from build123d import *

# Parameters (mm, degrees)
ESQUISSE2_W              = 92.64
ESQUISSE2_H              = 119.96
ESQUISSE2_W_2            = 88.74
ESQUISSE2_H_2            = 116.06
BASE_DEPTH               = 3
ESQUISSE3_R              = 4.5
SUPPORT_PCB_DEPTH        = 5
ESQUISSE4_R              = 2.25
ESQUISSE4_R_2            = 1.5
INSERT_M3_PCB_DEPTH      = 3
ESQUISSE4_3_R            = 1.5
PASSAGE_M3_PCB_DEPTH     = 5
ESQUISSE2_4_W            = 92.64
ESQUISSE2_4_H            = 119.96
ESQUISSE2_4_W_2          = 88.74
ESQUISSE2_4_H_2          = 116.06
WALLS_DEPTH              = 27
OUVERTURE_CONN_CMC_REACH = 133.396
ESQUISSE5_W              = 46.7
ESQUISSE5_H              = 20.1
CHANFREIN1_SIZE          = 12
CONG_1_R                 = 2
ESQUISSE6_R              = 2.25
INSERT_M3_BOX_DEPTH      = 3
ESQUISSE6_3_R            = 1.6
PASSAGE_M3_BOX_DEPTH     = 18
ESQUISSE10_R             = 3.1
BOSS_EXTRU_2_DEPTH       = 5
CONG_4_R                 = 5
PASSAGE_MAP_REACH        = 134.436
ESQUISSE11_R             = 3.5


with BuildPart() as part:
    # Esquisse2 → Base (new body)
    # profile 1 of 2: a face of its own
    with BuildSketch(Plane(origin=(0, 0, 0), x_dir=(1, 0, 0), z_dir=(0, 1, 0))):
        with Locations((0, 0.45)):
            Rectangle(ESQUISSE2_W, ESQUISSE2_H)
        with Locations((0, 0.45)):
            Rectangle(ESQUISSE2_W_2, ESQUISSE2_H_2, mode=Mode.SUBTRACT)
    # profile 2 of 2: a face of its own
    with BuildSketch(Plane(origin=(0, 0, 0), x_dir=(1, 0, 0), z_dir=(0, 1, 0))):
        with Locations((0, 0.45)):
            Rectangle(ESQUISSE2_W_2, ESQUISSE2_H_2)
    extrude(amount=-BASE_DEPTH)

    # Esquisse3 → Support_PCB (add)
    with BuildSketch(Plane(origin=(0, 0, 0), x_dir=(1, 0, 0), z_dir=(0, 1, 0))):
        with Locations(Location((-34.81, 28.71, 0), (0, 0, 270))):
            Circle(ESQUISSE3_R)
        with Locations(Location((34.79, 28.71, 0), (0, 0, 270))):
            Circle(ESQUISSE3_R)
        with Locations(Location((-19.57, -48, 0), (0, 0, 90))):
            Circle(ESQUISSE3_R)
        with Locations(Location((34.79, -48, 0), (0, 0, 90))):
            Circle(ESQUISSE3_R)
    extrude(amount=SUPPORT_PCB_DEPTH)

    # Esquisse4 → Insert_M3_PCB (cut)
    # profile 1 of 8: a face of its own
    with BuildSketch(Plane(origin=(0, 5, 0), x_dir=(1, 0, 0), z_dir=(0, 1, 0))):
        with Locations(Location((-34.81, 28.71, 0), (0, 0, 270))):
            Circle(ESQUISSE4_R)
        with Locations((-34.81, 28.71)):
            Circle(ESQUISSE4_R_2, mode=Mode.SUBTRACT)
    # profile 2 of 8: a face of its own
    with BuildSketch(Plane(origin=(0, 5, 0), x_dir=(1, 0, 0), z_dir=(0, 1, 0))):
        with Locations((-34.81, 28.71)):
            Circle(ESQUISSE4_R_2)
    # profile 3 of 8: a face of its own
    with BuildSketch(Plane(origin=(0, 5, 0), x_dir=(1, 0, 0), z_dir=(0, 1, 0))):
        with Locations(Location((34.79, 28.71, 0), (0, 0, 270))):
            Circle(ESQUISSE4_R)
        with Locations((34.79, 28.71)):
            Circle(ESQUISSE4_R_2, mode=Mode.SUBTRACT)
    # profile 4 of 8: a face of its own
    with BuildSketch(Plane(origin=(0, 5, 0), x_dir=(1, 0, 0), z_dir=(0, 1, 0))):
        with Locations((34.79, 28.71)):
            Circle(ESQUISSE4_R_2)
    # profile 5 of 8: a face of its own
    with BuildSketch(Plane(origin=(0, 5, 0), x_dir=(1, 0, 0), z_dir=(0, 1, 0))):
        with Locations(Location((34.79, -48, 0), (0, 0, 270))):
            Circle(ESQUISSE4_R)
        with Locations((34.79, -48)):
            Circle(ESQUISSE4_R_2, mode=Mode.SUBTRACT)
    # profile 6 of 8: a face of its own
    with BuildSketch(Plane(origin=(0, 5, 0), x_dir=(1, 0, 0), z_dir=(0, 1, 0))):
        with Locations((34.79, -48)):
            Circle(ESQUISSE4_R_2)
    # profile 7 of 8: a face of its own
    with BuildSketch(Plane(origin=(0, 5, 0), x_dir=(1, 0, 0), z_dir=(0, 1, 0))):
        with Locations(Location((-19.57, -48, 0), (0, 0, 270))):
            Circle(ESQUISSE4_R)
        with Locations((-19.57, -48)):
            Circle(ESQUISSE4_R_2, mode=Mode.SUBTRACT)
    # profile 8 of 8: a face of its own
    with BuildSketch(Plane(origin=(0, 5, 0), x_dir=(1, 0, 0), z_dir=(0, 1, 0))):
        with Locations((-19.57, -48)):
            Circle(ESQUISSE4_R_2)
    extrude(amount=-INSERT_M3_PCB_DEPTH, mode=Mode.SUBTRACT)

    # Esquisse4<3> → Passage M3_PCB (cut)
    with BuildSketch(Plane(origin=(0, 5, 0), x_dir=(1, 0, 0), z_dir=(0, 1, 0))):
        with Locations(Location((-19.57, -48, 0), (0, 0, 270))):
            Circle(ESQUISSE4_3_R)
        with Locations(Location((34.79, -48, 0), (0, 0, 270))):
            Circle(ESQUISSE4_3_R)
        with Locations(Location((34.79, 28.71, 0), (0, 0, 270))):
            Circle(ESQUISSE4_3_R)
        with Locations(Location((-34.81, 28.71, 0), (0, 0, 270))):
            Circle(ESQUISSE4_3_R)
    extrude(amount=-PASSAGE_M3_PCB_DEPTH, mode=Mode.SUBTRACT)

    # Esquisse2<4> → Walls (add)
    with BuildSketch(Plane(origin=(0, 0, 0), x_dir=(1, 0, 0), z_dir=(0, 1, 0))):
        with Locations((0, 0.45)):
            Rectangle(ESQUISSE2_4_W, ESQUISSE2_4_H)
        with Locations((0, 0.45)):
            Rectangle(ESQUISSE2_4_W_2, ESQUISSE2_4_H_2, mode=Mode.SUBTRACT)
    extrude(amount=WALLS_DEPTH)

    # Esquisse5 → Ouverture_Conn_CMC (cut, up to next)
    with BuildSketch(Plane(origin=(0, 0, -60.43), x_dir=(-1, 0, 0), z_dir=(0, 0, -1)), mode=Mode.PRIVATE) as ouverture_conn_cmc_sk1:
        with Locations((0, 16.95)):
            Rectangle(ESQUISSE5_W, ESQUISSE5_H)
    ouverture_conn_cmc_tool1 = extrude(ouverture_conn_cmc_sk1.sketch, amount=-OUVERTURE_CONN_CMC_REACH, mode=Mode.PRIVATE) & part.part
    add(ouverture_conn_cmc_tool1.solids().sort_by_distance((0, 16.95, -60.43))[0], mode=Mode.SUBTRACT)

    # Chanfrein1
    chanfrein1_edges = [part.edges().sort_by_distance(p)[0] for p in [
        (-44.37, 13.5, -58.48),
        (44.37, 13.5, -58.48),
        (44.37, 13.5, 57.58),
        (-44.37, 13.5, 57.58),
    ]]
    chamfer(chanfrein1_edges, length=CHANFREIN1_SIZE)

    # Congé1
    # the kernel refuses this fillet: 2 mm, written as the material it adds along each edge
    with BuildSketch(Plane(origin=(-37.37, 0, -58.48), x_dir=(0, 1, 0), z_dir=(1, 0, 0)), Plane(origin=(37.37, 0, 57.58), x_dir=(0, 1, 0), z_dir=(-1, 0, 0))) as cong_1_piece_1:
        with BuildLine():
            CenterArc((CONG_1_R, CONG_1_R), CONG_1_R, 180, 90)
            Line((0, CONG_1_R), (0, 0))
            Line((0, 0), (CONG_1_R, 0))
        make_face()
    extrude(amount=74.74)
    with BuildSketch(Plane(origin=(44.37, 0, -51.48), x_dir=(0, 1, 0), z_dir=(0, 0, 1)), Plane(origin=(-44.37, 0, 50.58), x_dir=(0, 1, 0), z_dir=(0, 0, -1))) as cong_1_piece_2:
        with BuildLine():
            CenterArc((CONG_1_R, CONG_1_R), CONG_1_R, 180, 90)
            Line((0, CONG_1_R), (0, 0))
            Line((0, 0), (CONG_1_R, 0))
        make_face()
    extrude(amount=102.06)
    with BuildSketch(Plane(origin=(-34.81, 0, -28.71), x_dir=(0, 0, 1), z_dir=(-1, 0, 0))) as cong_1_piece_3:
        with BuildLine():
            CenterArc((4.5 + CONG_1_R, CONG_1_R), CONG_1_R, 180, 90)
            Line((4.5, CONG_1_R), (4.5, 0))
            Line((4.5, 0), (4.5 + CONG_1_R, 0))
        make_face()
    revolve(axis=Axis((-34.81, 0, -28.71), (0, 1, 0)))
    with BuildSketch(Plane(origin=(34.79, 0, -28.71), x_dir=(0, 0, 1), z_dir=(-1, 0, 0))) as cong_1_piece_4:
        with BuildLine():
            CenterArc((4.5 + CONG_1_R, CONG_1_R), CONG_1_R, 180, 90)
            Line((4.5, CONG_1_R), (4.5, 0))
            Line((4.5, 0), (4.5 + CONG_1_R, 0))
        make_face()
    revolve(axis=Axis((34.79, 0, -28.71), (0, 1, 0)))
    with BuildSketch(Plane(origin=(-19.57, 0, 48), x_dir=(0, 0, -1), z_dir=(1, 0, 0))) as cong_1_piece_5:
        with BuildLine():
            CenterArc((4.5 + CONG_1_R, CONG_1_R), CONG_1_R, 180, 90)
            Line((4.5, CONG_1_R), (4.5, 0))
            Line((4.5, 0), (4.5 + CONG_1_R, 0))
        make_face()
    revolve(axis=Axis((-19.57, 0, 48), (0, 1, 0)))
    with BuildSketch(Plane(origin=(34.79, 0, 48), x_dir=(0, 0, -1), z_dir=(1, 0, 0))) as cong_1_piece_6:
        with BuildLine():
            CenterArc((4.5 + CONG_1_R, CONG_1_R), CONG_1_R, 180, 90)
            Line((4.5, CONG_1_R), (4.5, 0))
            Line((4.5, 0), (4.5 + CONG_1_R, 0))
        make_face()
    revolve(axis=Axis((34.79, 0, 48), (0, 1, 0)))
    # the kernel refuses this fillet: 2 mm, written as the material it takes off along each edge
    with BuildSketch(Plane(origin=(46.32, 32, -60.43), x_dir=(-1, 0, 0), z_dir=(0, -1, 0)), Plane(origin=(46.32, 32, 59.53), x_dir=(0, 0, -1), z_dir=(0, -1, 0)), Plane(origin=(-46.32, -8, -60.43), x_dir=(1, 0, 0), z_dir=(0, 1, 0))) as cong_1_2_piece_1:
        with BuildLine():
            CenterArc((CONG_1_R, -CONG_1_R), CONG_1_R, 90, 90)
            Line((0, -CONG_1_R), (0, 0))
            Line((0, 0), (CONG_1_R, 0))
        make_face()
    extrude(amount=40, mode=Mode.SUBTRACT)
    with BuildSketch(Plane(origin=(-46.32, -8, 59.53), x_dir=(1, 0, 0), z_dir=(0, 1, 0))) as cong_1_2_piece_2:
        with BuildLine():
            CenterArc((CONG_1_R, CONG_1_R), CONG_1_R, 180, 90)
            Line((0, CONG_1_R), (0, 0))
            Line((0, 0), (CONG_1_R, 0))
        make_face()
    extrude(amount=40, mode=Mode.SUBTRACT)

    # Esquisse6 → Insert_M3_Box (cut)
    with BuildSketch(Plane(origin=(0, 27, 0), x_dir=(1, 0, 0), z_dir=(0, 1, 0))):
        with Locations(Location((-41.248784258, 55.358784258, 0), (0, 0, 270))):
            Circle(ESQUISSE6_R)
        with Locations(Location((-41.248784258, -54.458784258, 0), (0, 0, 270))):
            Circle(ESQUISSE6_R)
        with Locations(Location((41.248784258, 55.358784258, 0), (0, 0, 270))):
            Circle(ESQUISSE6_R)
        with Locations(Location((41.248784258, -54.458784258, 0), (0, 0, 270))):
            Circle(ESQUISSE6_R)
    extrude(amount=-INSERT_M3_BOX_DEPTH, mode=Mode.SUBTRACT)

    # Esquisse6<3> → Passage_M3_Box (cut)
    with BuildSketch(Plane(origin=(0, 27, 0), x_dir=(1, 0, 0), z_dir=(0, 1, 0))):
        with Locations(Location((-41.248784258, 55.358784258, 0), (0, 0, 270))):
            Circle(ESQUISSE6_3_R)
        with Locations(Location((-41.248784258, -54.458784258, 0), (0, 0, 270))):
            Circle(ESQUISSE6_3_R)
        with Locations(Location((41.248784258, 55.358784258, 0), (0, 0, 270))):
            Circle(ESQUISSE6_3_R)
        with Locations(Location((41.248784258, -54.458784258, 0), (0, 0, 270))):
            Circle(ESQUISSE6_3_R)
    extrude(amount=-PASSAGE_M3_BOX_DEPTH, mode=Mode.SUBTRACT)

    # Esquisse10 → Boss.-Extru.2 (add)
    # profile 1 of 2: a face of its own
    with BuildSketch(Plane.XZ.offset(3)):
        with BuildLine():
            Line((46.32, 25), (66.32, 5))
            ThreePointArc((66.32, 5), (68.391067812, 0), (66.32, -5))
            Line((66.32, -5), (46.32, -25))
            Line((46.32, -25), (46.32, 25))
        make_face()
        with Locations(Location((58.32, 0, 0), (0, 0, 270))):
            Circle(ESQUISSE10_R, mode=Mode.SUBTRACT)
    # profile 2 of 2: a face of its own
    with BuildSketch(Plane.XZ.offset(3)):
        with BuildLine():
            Line((-46.32, 25), (-66.32, 5))
            ThreePointArc((-66.32, 5), (-68.391067812, 0), (-66.32, -5))
            Line((-66.32, -5), (-46.32, -25))
            Line((-46.32, -25), (-46.32, 25))
        make_face()
        with Locations(Location((-58.32, 0, 0), (0, 0, 90))):
            Circle(ESQUISSE10_R, mode=Mode.SUBTRACT)
    extrude(amount=-BOSS_EXTRU_2_DEPTH)

    # Congé4
    cong_4_edges = [part.edges().sort_by_distance(p)[0] for p in [
        (46.32, 2, 0),
        (46.32, -0.5, -25),
        (46.32, -0.5, 25),
        (-46.32, 2, 0),
        (-46.32, -0.5, 25),
        (-46.32, -0.5, -25),
    ]]
    fillet(cong_4_edges, radius=CONG_4_R)

    # Esquisse11 → Passage_MAP (cut, up to next)
    with BuildSketch(Plane(origin=(46.32, 0, 0), x_dir=(0, 0, -1), z_dir=(1, 0, 0)), mode=Mode.PRIVATE) as passage_map_sk1:
        with Locations((-14.53, 12.6)):
            Circle(ESQUISSE11_R)
    passage_map_tool1 = extrude(passage_map_sk1.sketch, amount=-PASSAGE_MAP_REACH, mode=Mode.PRIVATE) & part.part
    add(passage_map_tool1.solids().sort_by_distance((46.32, 12.6, 14.53))[0], mode=Mode.SUBTRACT)


solid = part.part
Design review of the part built by this model. Coordinates are the model's own, in mm. A direction names the side the tool comes from. Round coordinates to 2 decimals unless told otherwise and drop trailing zeros. Write each loop counter-clockwise with the first axis right and the second up, starting at its lowest first coordinate (ties: lowest second). Pieces come first, ordered by that corner, then holes.
Item 1: Draft analysis for pull direction X (two halves, no side actions). For faces 4 (the flat face through (-45, 27, -5)), 5 (the cylindrical face through (-68.39, -0.54, 0.08)), 6 (the flat face through (-1, 0, -1)), state which applies: released by +X, released by -X, zero draft, split by the parting line, or undercut.
Item 2: Consider section A-A on z = 14.53. Give the boundary of the cut face in (x, y).
Item 3: Consider section C-C on z = 0. Give the boundary of the cut face in (x, y).
Item 4: Consider section D-D on y = 22. Give the boundary of the cut face in (x, z).
Item 5: Consider section B-B on x = 58.32. Give the boundary of the cut face in (y, z), and give its area (3 significant figures).
Item 6: For pin 1 Ø3 at (x, z) = (31.5, 30) entering from +Y; pin 2 Ø6 at (y, z) = (12.5, 38.5) entering from -X; pin 3 Ø3 at (y, z) = (11.5, -22.5) entering from +X, all flat-tipped, find the tip position at first contact; note any pin that passes through.
Item 7: Wall thickness on L1, parallel to X at y = 3.05, z = -28.71; L2, parallel to X at y = 22, z = 6; L3, parallel to Z at x = 31.5, y = 26: over which ranges is each line inside the solid? List them lowest first.
Item 8: For faces 1 (the cylindrical face through (-34.74, 1.01, -30.21)), 2 (the cylindrical face through (45.36, 15.55, 12.65)), 3 (the flat face through (57.18, -0.53, -14.14)), list the 3-axis set-ups (+Z, -Z, +X, -X, +Y, -Y) from which the entire face can be reached by the end or side of a thin tool; tool diameter is ignored.
Check values:
1. face 4: zero draft
1. face 5: released by -X
1. face 6: undercut
2. outline: (-56.79, -3) - (56.79, -3) - (56.79, 2) - (51.32, 2) arc R5 cw to (46.32, 7) - (46.32, 9.1) - (44.37, 9.1) - (44.37, 2) arc R2 cw to (42.37, 0) - (-42.37, 0) arc R2 cw to (-44.37, 2) - (-44.37, 27) - (-46.32, 27) - (-46.32, 7) arc R5 cw to (-51.32, 2) - (-56.79, 2) - close; (44.37, 16.1) - (46.32, 16.1) - (46.32, 27) - (44.37, 27) - close
3. outline: (-68.39, -3) - (-61.42, -3) - (-61.42, 2) - (-68.39, 2) - close; (-55.22, -3) - (55.22, -3) - (55.22, 2) - (51.32, 2) arc R5 cw to (46.32, 7) - (46.32, 27) - (44.37, 27) - (44.37, 2) arc R2 cw to (42.37, 0) - (-42.37, 0) arc R2 cw to (-44.37, 2) - (-44.37, 27) - (-46.32, 27) - (-46.32, 7) arc R5 cw to (-51.32, 2) - (-55.22, 2) - close; (61.42, -3) - (68.39, -3) - (68.39, 2) - (61.42, 2) - close
4. outline: (-46.32, -58.43) arc R2 ccw to (-44.32, -60.43) - (-23.35, -60.43) - (-23.35, -58.48) - (-32.37, -58.48) - (-44.37, -46.48) - (-44.37, 45.58) - (-32.37, 57.58) - (32.37, 57.58) - (44.37, 45.58) - (44.37, -46.48) - (32.37, -58.48) - (23.35, -58.48) - (23.35, -60.43) - (44.32, -60.43) arc R2 ccw to (46.32, -58.43) - (46.32, 57.53) arc R2 ccw to (44.32, 59.53) - (-44.32, 59.53) arc R2 ccw to (-46.32, 57.53) - close; hole circle Ø3.2 at (-41.25, -55.36); hole circle Ø3.2 at (-41.25, 54.46); hole circle Ø3.2 at (41.25, -55.36); hole circle Ø3.2 at (41.25, 54.46)
5. outline: (-3, -13) - (2, -13) - (2, -3.1) - (-3, -3.1) - close; (-3, 3.1) - (2, 3.1) - (2, 13) - (-3, 13) - close
5. area: 99.0 mm2
6. pin 1: stops at y = 0
6. pin 2: stops at x = -46.32
6. pin 3: stops at x = 46.32
7. L1: x = -46.32 to -44.37, -39.31 to -37.06, -32.56 to -30.31, 30.29 to 32.54, 37.04 to 39.29, 44.37 to 46.32
7. L2: x = -46.32 to -44.37, 44.37 to 46.32
7. L3: z = -60.43 to -58.48, 57.58 to 59.53
8. face 1: +Y
8. face 2: +X
8. face 3: -Z, +X, +Y, -Y
